Answer from the drawing. Dimensions are ordinates in mm from the lowest x, y and z of the part. A direction names the side the tool comes from. Coordinates: 2 decimals unless noted, no trailing zeros. Write each loop counter-clockwise with the first axis right and the second up, starting at its lowest first coordinate (ties: lowest second). Pieces come first, ordered by that corner, then holes.
(1) Find the intervals of material crossed by probe 1 along X at (y, z) = (3.8, 2.25); probe 2 along X at (y, z) = (1.05, 2.5); probe 3 along Y at (x, z) = (6.25, 3.1), in increasing order.
(2) Section C-C on x = 7.5 is taken. Write down the section's boundary in (y, z), then the cut area to 3 significant figures.
(3) Section B-B on z = 2 is taken. Write down the section's boundary in (x, y), then the cut area to 3 significant figures.
(4) Section D-D on z = 0.6 is taken. Write down the section's boundary in (x, y).
(5) Given pin 1 (1.5 mm diameter, centred on x = 13, z = 0.5, fed in from +Y); pin 2 (1.6 mm diameter, centred on x = 2, z = 2, fed in from -Y), each flat-ended and moving along its own axis, determine where each tip first touches the part or whether it passes through.
(6) Which of the six approach directions +Z, -Z, +X, -X, +Y, -Y give full straight-line access (tool end or side, diameter ignored) to the marked faces 1, 2, 3, 4 and 5?
(7) Section A-A on y = 2 is taken. Write down the section's boundary in (x, z), then the cut area to 3 significant figures.
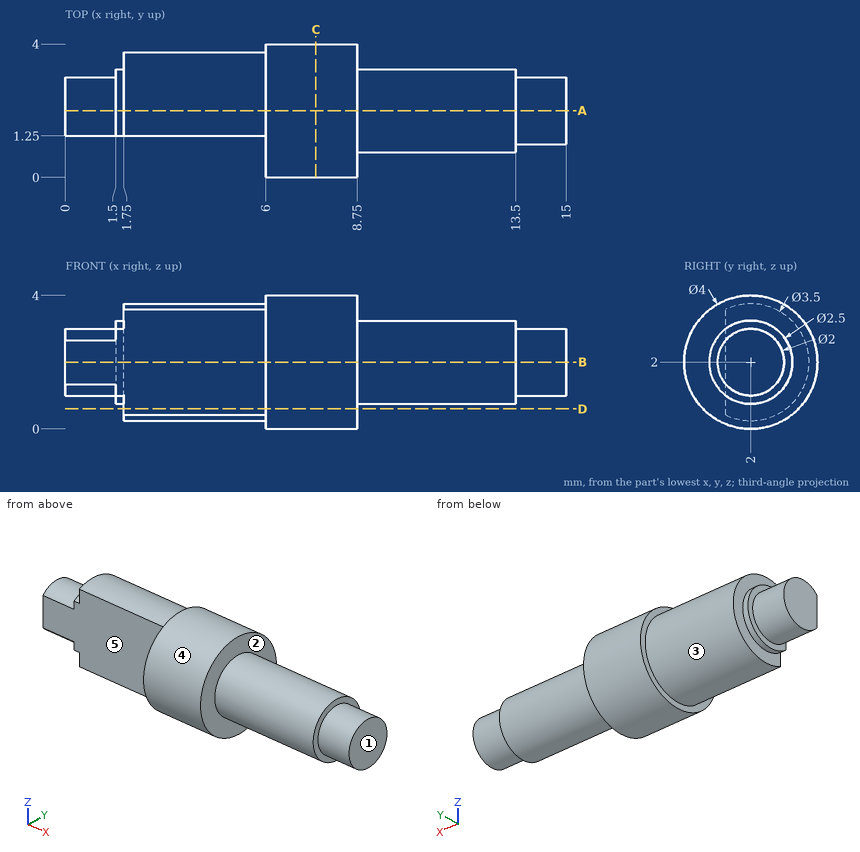
Response:
1. probe 1: x = 6 to 8.75
1. probe 2: x = 6 to 13.5
1. probe 3: y = 0.33 to 3.67
2. outline: circle Ø4 at (2, 2)
2. area: 12.6 mm2
3. outline: (0, 1.25) - (6, 1.25) - (6, 0) - (8.75, 0) - (8.75, 0.75) - (13.5, 0.75) - (13.5, 1) - (15, 1) - (15, 3) - (13.5, 3) - (13.5, 3.25) - (8.75, 3.25) - (8.75, 4) - (6, 4) - (6, 3.75) - (1.75, 3.75) - (1.75, 3.25) - (1.5, 3.25) - (1.5, 3) - (0, 3) - close
3. area: 39.6 mm2
4. outline: (1.75, 1.25) - (6, 1.25) - (6, 0.57) - (8.75, 0.57) - (8.75, 3.43) - (6, 3.43) - (6, 3.05) - (1.75, 3.05) - close
5. pin 1: stops at y = 3
5. pin 2: stops at y = 1.25
6. face 1: +Z, -Z, +X, +Y, -Y
6. face 2: +X
6. face 3: -X
6. face 4: +X, -X
6. face 5: +Z, -Z, -X, -Y
7. outline: (0, 1) - (1.5, 1) - (1.5, 0.75) - (1.75, 0.75) - (1.75, 0.25) - (6, 0.25) - (6, 0) - (8.75, 0) - (8.75, 0.75) - (13.5, 0.75) - (13.5, 1) - (15, 1) - (15, 3) - (13.5, 3) - (13.5, 3.25) - (8.75, 3.25) - (8.75, 4) - (6, 4) - (6, 3.75) - (1.75, 3.75) - (1.75, 3.25) - (1.5, 3.25) - (1.5, 3) - (0, 3) - close
7. area: 44.4 mm2
